Part model, mm, in its own coordinate system. A direction names the side the tool comes from. Coordinates: 2 decimals unless noted, no trailing zeros. Order: outer loops, then holes, each group sorted by start corner. A loop starts at its lowest first (then second) coordinate and runs counter-clockwise, first axis right, second up.
1) Cut at B-B (z = -1.25). List the corners of the cut face in (x, y).
2) Pin check, flat tips, straight feed: pin 1 Ø2 at (x, z) = (-26, -17.5) entering from -Y; pin 2 Ø4 at (x, z) = (-3, -3) entering from +Y; pin 3 Ø1.5 at (x, y) = (-19.5, 13.5) entering from -Z. Stop position of each tip, or through.
3) Cut at D-D (z = -16). List the corners of the cut face in (x, y).
4) Wall check: L1, parallel to Z at x = -27, y = 3.3; L2, parallel to X at y = 10.5, z = -17.5; L3, parallel to Z at x = -8.75, y = 6. Give the ranges that are in metal, low to high.
5) Mould opens along X. For faces 5 (the flat face through (-3, 36, -17)), 6 (the flat face through (-27, 20, -20)), 7 (the flat face through (-30, 21, -10)) say: +X half, -X half, draft (parallel to the pull), parting line (faces both ways), or undercut.
6) Cut at A-A (x = -27). List the corners of the cut face in (y, z), and give its area (3 significant figures).
7) Cut at C-C (y = 12). List the corners of the cut face in (x, z), and give its area (3 significant figures).
8) Tool access for faces 1 (the flat face through (-7, 20, -2)), 2 (the flat face through (-27, 36, -3)), 3 (the flat face through (-7, 20, -19)), 4 (the flat face through (-27, 5, -3)): list every direction of +Z, -Z, +X, -X, +Y, -Y with a clear straight run to the whole face (end or side of a thin tool).
```python
from build123d import *

# Parameters (mm, degrees)
SKETCH_1_W           = 30
SKETCH_1_H           = 20
EXTRUDE_1_DEPTH      = 41
CUT_EXTRUDE_15_REACH = 56.599
SKETCH_17_W          = 7
SKETCH_17_H          = 8
SKETCH_17_W_2        = 16
SKETCH_17_H_2        = 3
SKETCH_20_R          = 2.25
CUT_EXTRUDE_18_DEPTH = 5
SKETCH_21_W          = 8
SKETCH_21_H          = 41
EXTRUDE_2_DEPTH      = 7
SKETCH_22_W          = 8
SKETCH_22_H          = 41
EXTRUDE_3_DEPTH      = 7
CUT_EXTRUDE_START    = -5
SKETCH_23_R          = 2.25
CUT_EXTRUDE_19_DEPTH = 5


with BuildPart() as part:
    # 草图1 → 凸台-拉伸1 (new body)
    with BuildSketch(Plane(origin=(0, 0, 0), x_dir=(1, 0, 0), z_dir=(0, 1, 0))):
        with Locations((-15, 10)):
            Rectangle(SKETCH_1_W, SKETCH_1_H)
    extrude(amount=EXTRUDE_1_DEPTH)

    # 草图17 → 切除-拉伸15 (cut, up to next)
    with BuildSketch(Plane.XZ, mode=Mode.PRIVATE) as cut_extrude_15_sk1:
        with Locations((-26.5, -10)):
            Rectangle(SKETCH_17_W, SKETCH_17_H)
    cut_extrude_15_tool1 = extrude(cut_extrude_15_sk1.sketch, amount=-CUT_EXTRUDE_15_REACH, mode=Mode.PRIVATE) & part.part
    # 草图17 → 切除-拉伸15 (cut, up to next)
    with BuildSketch(Plane.XZ, mode=Mode.PRIVATE) as cut_extrude_15_sk2:
        with Locations((-3.5, -10)):
            Rectangle(SKETCH_17_W, SKETCH_17_H)
    cut_extrude_15_tool2 = extrude(cut_extrude_15_sk2.sketch, amount=-CUT_EXTRUDE_15_REACH, mode=Mode.PRIVATE) & part.part
    # 草图17 → 切除-拉伸15 (cut, up to next)
    with BuildSketch(Plane.XZ, mode=Mode.PRIVATE) as cut_extrude_15_sk3:
        with Locations((-15, -1.5)):
            Rectangle(SKETCH_17_W_2, SKETCH_17_H_2)
    cut_extrude_15_tool3 = extrude(cut_extrude_15_sk3.sketch, amount=-CUT_EXTRUDE_15_REACH, mode=Mode.PRIVATE) & part.part
    # 草图17 → 切除-拉伸15 (cut, up to next)
    with BuildSketch(Plane.XZ, mode=Mode.PRIVATE) as cut_extrude_15_sk4:
        with Locations((-15, -18.5)):
            Rectangle(SKETCH_17_W_2, SKETCH_17_H_2)
    cut_extrude_15_tool4 = extrude(cut_extrude_15_sk4.sketch, amount=-CUT_EXTRUDE_15_REACH, mode=Mode.PRIVATE) & part.part
    add(cut_extrude_15_tool1.solids().sort_by_distance((-26.5, 0, -10))[0], mode=Mode.SUBTRACT)
    add(cut_extrude_15_tool2.solids().sort_by_distance((-3.5, 0, -10))[0], mode=Mode.SUBTRACT)
    add(cut_extrude_15_tool3.solids().sort_by_distance((-15, 0, -1.5))[0], mode=Mode.SUBTRACT)
    add(cut_extrude_15_tool4.solids().sort_by_distance((-15, 0, -18.5))[0], mode=Mode.SUBTRACT)

    # 草图20 → 切除-拉伸18 (cut)
    with BuildSketch(Plane(origin=(0, 41, 0), x_dir=(1, 0, 0), z_dir=(0, 1, 0))):
        with Locations(Location((-27, 17, 0), (0, 0, 270))):
            Circle(SKETCH_20_R)
        with Locations(Location((-27, 3, 0), (0, 0, 270))):
            Circle(SKETCH_20_R)
        with Locations(Location((-3, 3, 0), (0, 0, 270))):
            Circle(SKETCH_20_R)
        with Locations(Location((-3, 17, 0), (0, 0, 270))):
            Circle(SKETCH_20_R)
    extrude(amount=-CUT_EXTRUDE_18_DEPTH, mode=Mode.SUBTRACT)

    # 草图21 → 凸台-拉伸2 (add)
    with BuildSketch(Plane(origin=(-7, 0, 0), x_dir=(0, 0, -1), z_dir=(1, 0, 0))):
        with Locations((10, 20.5)):
            Rectangle(SKETCH_21_W, SKETCH_21_H)
    extrude(amount=EXTRUDE_2_DEPTH)

    # 草图22 → 凸台-拉伸3 (add)
    with BuildSketch(Plane.ZY.offset(23)):
        with Locations((-10, 20.5)):
            Rectangle(SKETCH_22_W, SKETCH_22_H)
    extrude(amount=EXTRUDE_3_DEPTH)

    # 草图23 → 切除-拉伸19 (cut)
    with BuildSketch(Plane.XZ.offset(CUT_EXTRUDE_START)):
        with Locations(Location((-3, -17, 0), (0, 0, 90))):
            Circle(SKETCH_23_R)
        with Locations(Location((-27, -17, 0), (0, 0, 90))):
            Circle(SKETCH_23_R)
        with Locations(Location((-27, -3, 0), (0, 0, 90))):
            Circle(SKETCH_23_R)
        with Locations(Location((-3, -3, 0), (0, 0, 90))):
            Circle(SKETCH_23_R)
    extrude(amount=CUT_EXTRUDE_19_DEPTH, mode=Mode.SUBTRACT)


solid = part.part
```
Geometry check:
1. outline: (-30, 0) - (-28.41, 0) - (-28.41, 5) - (-25.59, 5) - (-25.59, 0) - (-23, 0) - (-23, 41) - (-25.59, 41) - (-25.59, 36) - (-28.41, 36) - (-28.41, 41) - (-30, 41) - close; (-7, 0) - (-4.41, 0) - (-4.41, 5) - (-1.59, 5) - (-1.59, 0) - (0, 0) - (0, 41) - (-1.59, 41) - (-1.59, 36) - (-4.41, 36) - (-4.41, 41) - (-7, 41) - close
2. pin 1: stops at y = 5
2. pin 2: stops at y = 36
2. pin 3: stops at z = -17
3. outline: (-30, 0) - (-29.02, 0) - (-29.02, 5) - (-24.98, 5) - (-24.98, 0) - (-5.02, 0) - (-5.02, 5) - (-0.98, 5) - (-0.98, 0) - (0, 0) - (0, 41) - (-0.98, 41) - (-0.98, 36) - (-5.02, 36) - (-5.02, 41) - (-24.98, 41) - (-24.98, 36) - (-29.02, 36) - (-29.02, 41) - (-30, 41) - close
4. L1: z = -20 to -19.25, -14.75 to -5.25, -0.75 to 0
4. L2: x = -30 to -23, -7 to 0
4. L3: z = -17 to -3
5. face 5: undercut
5. face 6: draft
5. face 7: -X half
6. outline: (0, -20) - (41, -20) - (41, -19.25) - (36, -19.25) - (36, -14.75) - (41, -14.75) - (41, -5.25) - (36, -5.25) - (36, -0.75) - (41, -0.75) - (41, 0) - (0, 0) - (0, -0.75) - (5, -0.75) - (5, -5.25) - (0, -5.25) - (0, -14.75) - (5, -14.75) - (5, -19.25) - (0, -19.25) - close
6. area: 730 mm2
7. outline: (-30, -20) - (-23, -20) - (-23, -17) - (-7, -17) - (-7, -20) - (0, -20) - (0, 0) - (-7, 0) - (-7, -3) - (-23, -3) - (-23, 0) - (-30, 0) - close
7. area: 504 mm2
8. face 1: +Z, +Y, -Y
8. face 2: +Y
8. face 3: -Z, +Y, -Y
8. face 4: -Y
